Check sheet for the modelled part. Datum: model origin and axes. Units: mm. Face numbers are marked on the shaded views. A direction names the side the tool comes from. Give positions to 0.01 mm unless a question says otherwise; leave off trailing zeros. Order: outer loops, then holes, each group sorted by start corner. A loop starts at its lowest first (then second) coordinate and runs counter-clockwise, first axis right, second up. Notation, with made-up numbers: (55.5, -25) -> (86.5, -25) arc R15 ccw to (86.5, -17) -> close; hole circle Ø7 at (-12, 19). An arc over 180 degrees is marked (long way). Answer in a Markdown table with one row per item. Add a question column.
(1) Cross-section at C-C (y = -0.25). Record the cut outline in (x, z).
(2) Thickness scan on L1, parallel to Z at x = -4, y = 1.5; L2, parallel to Z at x = -7.5, y = 1; L3, parallel to Y at x = -6.25, z = 3. Record the ranges inside material, lowest first. Write a range as [from, to].
(3) Go/stop test with flat-tipped pins: pin 1 (6 mm diameter, centred on y = 1, z = 4.5, fed in from -X); pin 2 (3 mm diameter, centred on x = -4.5, y = 0, fed in from -Z); pin 3 (8.5 mm diameter, centred on x = -4, y = -0.5, fed in from +Z). Record where each tip stops, or that it passes through.
(4) Release check for a two-part mould opening along X. For the marked faces 1, 2, 3 and 4 record: released by +X, released by -X, zero draft, split by the parting line, or undercut.
(5) Cross-section at A-A (z = -1.75). Record the cut outline in (x, y), then the cut area to 3 significant figures.
(6) Set-up check for the marked faces 5, 6 and 7: record each of +Z, -Z, +X, -X, +Y, -Y from which the full face is reachable in a straight line by a thin tool's end or side.
(7) Cross-section at D-D (x = -3). Record the cut outline in (y, z), then the cut area to 3 significant figures.
(8) Cross-section at B-B (x = -10.75). Record the cut outline in (y, z).
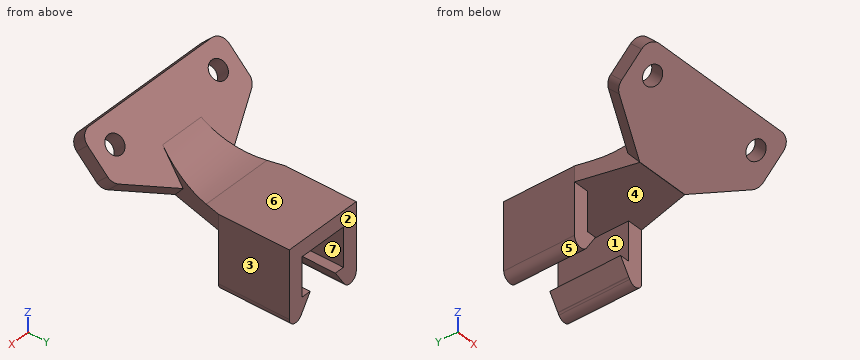
```python
from build123d import *

# Parameters (mm, degrees)
SKETCH2_W           = 8.999610642
SKETCH2_H           = 9.2
BOSS_EXTRUDE1_DEPTH = 2
BOSS_EXTRUDE2_START = 6.4
SKETCH3_W           = 8.999610642
SKETCH3_H           = 9.2
BOSS_EXTRUDE2_DEPTH = 2
SKETCH4_W           = 1.999805321
SKETCH4_H           = 9.2
BOSS_EXTRUDE3_DEPTH = 7
CUT_EXTRUDE2_DEPTH  = 9.2
BOSS_EXTRUDE4_DEPTH = 9.2
FILLET1_R           = 1
BOSS_EXTRUDE6_DEPTH = 1.999805321
SKETCH11_R          = 1.2
BOSS_EXTRUDE7_DEPTH = 2
FILLET2_R           = 10
SKETCH13_W          = 7
SKETCH13_H          = 0.042993575
BOSS_EXTRUDE8_DEPTH = 1


with BuildPart() as part:
    # Sketch2 → Boss-Extrude1 (new body)
    with BuildSketch(Plane(origin=(0, 0, 0), x_dir=(0, 0, -1), z_dir=(1, 0, 0))):
        Rectangle(SKETCH2_W, SKETCH2_H)
    extrude(amount=BOSS_EXTRUDE1_DEPTH)



with BuildPart() as body_2:
    # Sketch3 → Boss-Extrude2 (new body)
    with BuildSketch(Plane.ZY.offset(BOSS_EXTRUDE2_START)):
        Rectangle(SKETCH3_W, SKETCH3_H)
    extrude(amount=BOSS_EXTRUDE2_DEPTH)


with BuildPart() as part_1:
    add(part.part)

    add(body_2.part)  # Boss-Extrude3 merges body 2
    # Sketch4 → Boss-Extrude3 (add)
    with BuildSketch(Plane.ZY):
        with Locations((3.499902661, 0)):
            Rectangle(SKETCH4_W, SKETCH4_H)
    extrude(amount=BOSS_EXTRUDE3_DEPTH)

    # Sketch5 → Cut-Extrude2 (cut)
    with BuildSketch(Plane(origin=(0, 4.6, 0), x_dir=(1, 0, 0), z_dir=(0, 1, 0))):
        Polygon((-5.15, 2.55), (-1.25, 2.55), (0, 4.473076923), (0, 4.499805321), (0.017373458, 4.499805321), (2, 7.55), (-8.4, 7.55), (-6.417373458, 4.499805321), (-6.4, 4.499805321), (-6.4, 4.473076923), align=None)
        Polygon((0, 4.499805321), (0, 4.473076923), (0.017373458, 4.499805321), align=None)
        Polygon((-6.417373458, 4.499805321), (-6.4, 4.473076923), (-6.4, 4.499805321), align=None)
    extrude(amount=-CUT_EXTRUDE2_DEPTH, mode=Mode.SUBTRACT)

    # Sketch5<3> → Boss-Extrude4 (add)
    with BuildSketch(Plane(origin=(0, 4.6, 0), x_dir=(1, 0, 0), z_dir=(0, 1, 0))):
        Polygon((-6.4, 2.55), (-5.15, 2.55), (-6.4, 4.473076923), align=None)
        Polygon((-8.4, 4.499805321), (-6.417373458, 4.499805321), (-8.4, 7.55), align=None)
        Polygon((-1.25, 2.55), (0, 2.55), (0, 4.473076923), align=None)
        Polygon((0.017373458, 4.499805321), (2, 4.499805321), (2, 7.55), align=None)
    extrude(amount=-BOSS_EXTRUDE4_DEPTH)

    # Fillet1
    fillet1_edges = [part_1.edges().sort_by_distance(p)[0] for p in [
        (-8.4, 0, -7.55),
        (2, 0, -7.55),
    ]]
    fillet(fillet1_edges, radius=FILLET1_R)

    # Sketch9 → Boss-Extrude6 (add)
    with BuildSketch(Plane.XY.offset(4.499805321)):
        Polygon((-6.7, -11.6), (0.3, -11.6), (2, -4.6), (-8.4, -4.6), align=None)
    extrude(amount=-BOSS_EXTRUDE6_DEPTH)

    # Sketch11 → Boss-Extrude7 (add)
    with BuildSketch(Plane(origin=(0, -4.596209487, -4.559766639), x_dir=(1, 0, 0), z_dir=(0, 0.7099156022207138, 0.7042867581628958))):
        with BuildLine():
            Line((7.8, -19.262920267), (7.8, -15.587764453))
            ThreePointArc((7.8, -15.587764453), (7.614381512, -14.864991154), (7.103465011, -14.321097971))
            Line((7.103465011, -14.321097971), (0.3, -10.005560954))
            Line((0.3, -10.005560954), (-6.7, -10.005560954))
            Line((-6.7, -10.005560954), (-13.503465011, -14.321097971))
            ThreePointArc((-13.503465011, -14.321097971), (-14.014381512, -14.864991154), (-14.2, -15.587764453))
            Line((-14.2, -15.587764453), (-14.2, -19.262920267))
            ThreePointArc((-14.2, -19.262920267), (-13.760660172, -20.323580438), (-12.7, -20.762920267))
            Line((-12.7, -20.762920267), (6.3, -20.762920267))
            ThreePointArc((6.3, -20.762920267), (7.360660172, -20.323580438), (7.8, -19.262920267))
        make_face()
        with Locations(Location((4.825, -17.762920267, 0), (0, 0, 270))):
            Circle(SKETCH11_R, mode=Mode.SUBTRACT)
        with Locations(Location((-11.225, -17.762920267, 0), (0, 0, 270))):
            Circle(SKETCH11_R, mode=Mode.SUBTRACT)
    extrude(amount=BOSS_EXTRUDE7_DEPTH)

    # Fillet2
    fillet2_edges = [part_1.edges().sort_by_distance(p)[0] for p in [
        (-3.2, -10.766712787, 4.499805321),
    ]]
    fillet(fillet2_edges, radius=FILLET2_R)

    # Sketch13 → Boss-Extrude8 (add)
    with BuildSketch(Plane(origin=(0, 0, 2.5), x_dir=(-1, 0, 0), z_dir=(0, 0, -1))):
        with Locations((3.2, -11.621496787)):
            Rectangle(SKETCH13_W, SKETCH13_H)
    extrude(amount=-BOSS_EXTRUDE8_DEPTH)


solid = part_1.part
```
Answer below:
| question | item | result |
|---|---|---|
| 1 | outline | (-8.4, -4.18) arc R1 ccw to (-6.56, -4.72) -> (-5.15, -2.55) -> (-6.4, -2.55) -> (-6.4, 2.5) -> (0, 2.5) -> (0, -2.55) -> (-1.25, -2.55) -> (0.16, -4.72) arc R1 ccw to (2, -4.18) -> (2, 4.5) -> (-8.4, 4.5) -> close |
| 2 | L1 | z = [2.5, 4.5] |
| 2 | L2 | z = [-5.17, 4.5] |
| 2 | L3 | y = [-12.1, 4.6] |
| 3 | pin 1 | stops at x = -8.4 |
| 3 | pin 2 | stops at z = -3.86 |
| 3 | pin 3 | stops at z = 4.5 |
| 4 | face 1 | undercut |
| 4 | face 2 | zero draft |
| 4 | face 3 | released by +X |
| 4 | face 4 | undercut |
| 5 | outline | (-8.4, -4.6) -> (-6.4, -4.6) -> (-6.4, 4.6) -> (-8.4, 4.6) -> close; (0, -4.6) -> (2, -4.6) -> (2, 4.6) -> (0, 4.6) -> close |
| 5 | area | 36.8 mm² |
| 6 | face 5 | -Z, +Y, -Y |
| 6 | face 6 | +Z, +X, -X, +Y |
| 6 | face 7 | +Y, -Y |
| 7 | outline | (-19.22, 10.18) -> (-11.64, 2.54) -> (-11.64, 2.5) -> (4.6, 2.5) -> (4.6, 4.5) -> (-6.6, 4.5) arc R10 cw to (-13.7, 7.46) -> (-17.8, 11.59) -> close |
| 7 | area | 54.6 mm² |
| 8 | outline | (-19.22, 10.18) -> (-17.88, 8.83) -> (-16.46, 10.24) -> (-17.8, 11.59) -> close; (-16.33, 7.27) -> (-13.45, 4.37) -> (-12.03, 5.78) -> (-14.91, 8.68) -> close |
